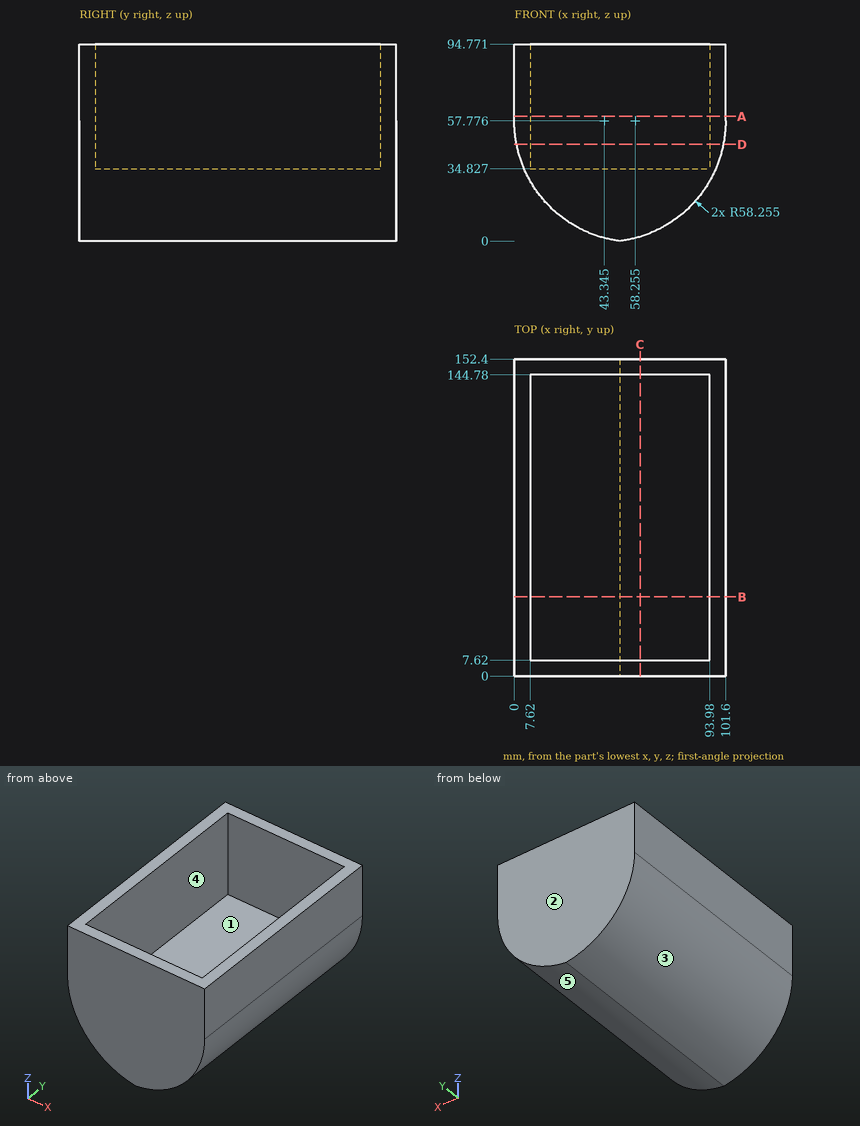
Drawing for the job (mm, zero at the part's lowest x, y, z). A direction names the side the tool comes from. Give positions to 0.01 mm unless a question says otherwise; leave off trailing zeros. Loops run counter-clockwise (first coordinate to the right, second up) from the corner with the lowest first, then second, coordinate; pieces in that order, holes last.
Item 1: Which spindle directions (+Z, -Z, +X, -X, +Y, -Y) get a long thin tool onto all of the face, cutting with end or side? Do the marked faces 4 and 5. Say none if no direction does.
Check values:
face 4: +Z
face 5: -Z, +X, +Y, -Y
Item 2: Slice it at D-D (z = 46.5). Write the cut outline in (x, y), plus the area to 3 significant figures.
Check values:
outline: (1.1, 0) - (100.5, 0) - (100.5, 152.4) - (1.1, 152.4) - close; hole (7.62, 7.62) - (93.98, 7.62) - (93.98, 144.78) - (7.62, 144.78) - close
area: 3,300 mm2
Item 3: Slice it at A-A (z = 60). Write the cut outline in (x, y).
Check values:
outline: (0, 0) - (101.6, 0) - (101.6, 152.4) - (0, 152.4) - close; hole (7.62, 7.62) - (93.98, 7.62) - (93.98, 144.78) - (7.62, 144.78) - close
Item 4: Slice it at B-B (y = 38). Write the cut outline in (x, z) (3 decimals), plus the area to 3 significant figures.
Check values:
outline: (0, 57.776) arc R58.255 ccw to (50.8, 0) arc R58.255 ccw to (101.6, 57.776) - (101.6, 94.771) - (93.98, 94.771) - (93.98, 34.827) - (7.62, 34.827) - (7.62, 94.771) - (0, 94.771) - close
area: 3,050 mm2
Item 5: Slice it at C-C (x = 60.5). Write the cut outline in (y, z), plus the area to 3 significant figures.
Check values:
outline: (0, 2.1) - (152.4, 2.1) - (152.4, 94.77) - (144.78, 94.77) - (144.78, 34.83) - (7.62, 34.83) - (7.62, 94.77) - (0, 94.77) - close
area: 5,900 mm2
Item 6: Drill centre lines: line 1 along Y through (x, z) = (88, 57.5); line 2 along X through (y, z) = (114, 88); line 3 along X through (y, z) = (113, 29). Where is each one in solid material? Low to high.
Check values:
line 1: y = 0 to 7.62, 144.78 to 152.4
line 2: x = 0 to 7.62, 93.98 to 101.6
line 3: x = 7.6 to 94
Item 7: Mould opens along X. For the marked faces 1, 2 and 3 say: +X half, -X half, draft (parallel to the pull), parting line (faces both ways), or undercut.
Check values:
face 1: undercut
face 2: draft
face 3: -X half
Item 8: Drop flat-ended pins along their axis: P1, Ø1.5, axis at x = 12.5, y = 130, coming from the +Z side; P2, Ø1, axis at x = 41, y = 133.5, coming from the -Z side; P3, Ø1.5, axis at x = 38.5, y = 129.5, coming from the -Z side. Give the stop position or say it passes through.
Check values:
P1: stops at z = 34.83
P2: stops at z = 1.98
P3: stops at z = 2.71
